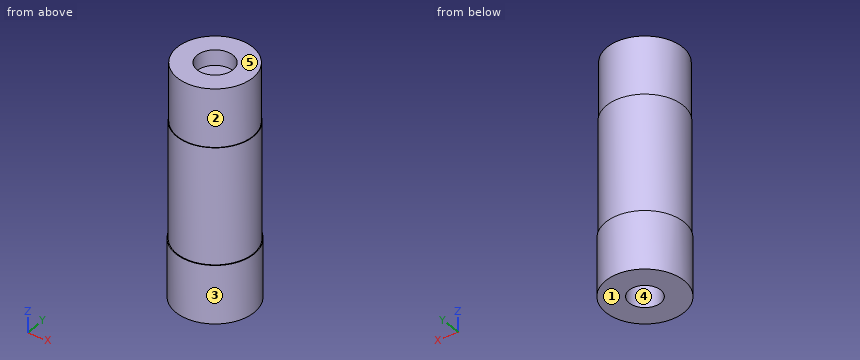
from build123d import *

# Parameters (mm, degrees)
SKETCH1_R           = 6.75
SKETCH1_R_2         = 2.725
BOSS_EXTRUDE2_DEPTH = 10
SKETCH2_R           = 6.6
BOSS_EXTRUDE3_DEPTH = 30
CUT_EXTRUDE1_START  = -10
SKETCH3_R           = 6.6
SKETCH3_R_2         = 6.5
CUT_EXTRUDE1_DEPTH  = 10
SKETCH4_R           = 3.1
CUT_EXTRUDE3_DEPTH  = 2.65


with BuildPart() as part:
    # Sketch1 → Boss-Extrude2 (new body)
    with BuildSketch(Plane.XY):
        Circle(SKETCH1_R)
        Circle(SKETCH1_R_2, mode=Mode.SUBTRACT)
    extrude(amount=BOSS_EXTRUDE2_DEPTH)

    # Sketch2 → Boss-Extrude3 (add)
    with BuildSketch(Plane.XY.offset(10)):
        Circle(SKETCH2_R)
    extrude(amount=BOSS_EXTRUDE3_DEPTH)

    # Sketch3 → Cut-Extrude1 (cut)
    with BuildSketch(Plane.XY.offset(40).offset(CUT_EXTRUDE1_START)):
        Circle(SKETCH3_R)
        Circle(SKETCH3_R_2, mode=Mode.SUBTRACT)
    extrude(amount=CUT_EXTRUDE1_DEPTH, mode=Mode.SUBTRACT)

    # Sketch4 → Cut-Extrude3 (cut)
    with BuildSketch(Plane.XY.offset(40)):
        Circle(SKETCH4_R)
    extrude(amount=-CUT_EXTRUDE3_DEPTH, mode=Mode.SUBTRACT)


solid = part.part
Geometry: final body of the model. Coordinates: model frame, mm. Face numbers are marked on the shaded views. A direction names the side the tool comes from. Coordinates: 2 decimals unless noted, no trailing zeros. Order: outer loops, then holes, each group sorted by start corner. A loop starts at its lowest first (then second) coordinate and runs counter-clockwise, first axis right, second up.
(1) Section query D-D (z = 20.5). Return the cut outline in (x, y).
(2) First-contact query: pin 1 (8 mm diameter, centred on y = 5, z = 27.5, fed in from +X); pin 2 (1.5 mm diameter, centred on y = -2, z = 17, fed in from -X); pin 3 (2 mm diameter, centred on y = -3, z = 34, fed in from -X). Flat tips, straight axial feed; report the tip coordinate or a pass-through.
(3) Access query for the marked faces 1 and 2. Directions: +Z, -Z, +X, -X, +Y, -Y. A direction counts if a zero-diameter tool reaches every point of the face in a straight line with its end or side. Return the directions, or none.
(4) Section query A-A (x = 0). Return the cut outline in (y, z) (3 decimals), plus the area to 3 significant figures.
(5) Section query C-C (z = 9.5). Return the cut outline in (x, y) (3 decimals).
(6) Material intervals for probe 1 along Y at (x, z) = (0, 39.25); probe 2 along Y at (x, z) = (0, 4.5) (3 decimals); probe 3 along Z at (x, y) = (5, 4.25), sorted ascending.
(7) Draft query along Y for the marked faces 3, 4 and 5. Return one class per face: pulls with the +Y half, pulls with the -Y half, needs draft (parallel to the pull), parting line crosses it, or undercut.
Solution:
1. outline: circle Ø13.2 at (0, 0)
2. pin 1: stops at x = 6.52
2. pin 2: stops at x = -6.48
2. pin 3: stops at x = -6.18
3. face 1: -Z, +X, -X, +Y, -Y
3. face 2: +Z
4. outline: (-6.75, 0) - (-2.725, 0) - (-2.725, 10) - (2.725, 10) - (2.725, 0) - (6.75, 0) - (6.75, 10) - (6.6, 10) - (6.6, 30) - (6.5, 30) - (6.5, 40) - (3.1, 40) - (3.1, 37.35) - (-3.1, 37.35) - (-3.1, 40) - (-6.5, 40) - (-6.5, 30) - (-6.6, 30) - (-6.6, 10) - (-6.75, 10) - close
4. area: 458 mm2
5. outline: circle Ø13.5 at (0, 0); hole circle Ø5.45 at (0, 0)
6. probe 1: y = -6.5 to -3.1, 3.1 to 6.5
6. probe 2: y = -6.75 to -2.725, 2.725 to 6.75
6. probe 3: z = 0 to 30
7. face 3: parting line crosses it
7. face 4: undercut
7. face 5: needs draft
